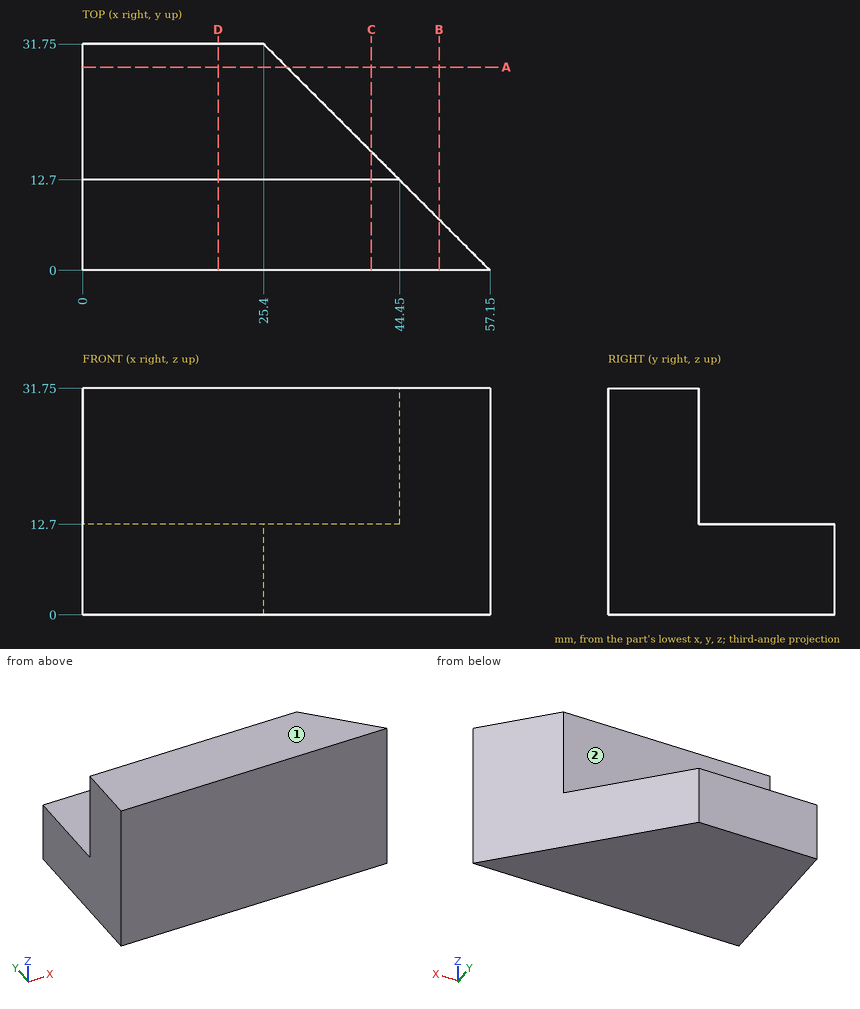
Can you work these out from the drawing? Everything is in mm from the part's minimum corner. A direction names the side the tool comes from. Coordinates: 2 decimals unless noted, no trailing zeros. Write each loop counter-clockwise with the first axis right and the second up, starting at its lowest first coordinate (ties: lowest second). Pieces come first, ordered by that corner, then holes. Notation, with made-up numbers: (-8.75, 32) -> (1.25, 32) arc R14 ccw to (1.25, 49) -> close; hole circle Ø11 at (76.5, -39.5). An arc over 180 degrees is marked (long way). Return JSON: item names as keys, results as strings.
(1) Imagine slicing it at B-B, the plane x = 50. Please give me the cut outline in (y, z), then the cut area to 3 significant figures.
Numbers:
{"outline": "(0, 0) -> (7.15, 0) -> (7.15, 31.75) -> (0, 31.75) -> close", "area": "227 mm2"}
(2) I need wall thicknesses on L1, parallel to Z at x = 5, y = 13; L2, parallel to X at y = 12, z = 20. Which ranges of each line are inside material? Lowest first, please.
Numbers:
{"L1": "z = 0 to 12.7", "L2": "x = 0 to 45.15"}
(3) Imagine slicing it at C-C, the plane x = 40.5. Please give me the cut outline in (y, z).
Numbers:
{"outline": "(0, 0) -> (16.65, 0) -> (16.65, 12.7) -> (12.7, 12.7) -> (12.7, 31.75) -> (0, 31.75) -> close"}
(4) Which directions (+Z, -Z, +X, -X, +Y, -Y) give clear straight access to the entire face, cutting with the end or side of a thin tool? Please do the marked faces 1 and 2.
Numbers:
{"face 1": "+Z, +X, -X, +Y, -Y", "face 2": "+Z, +X, -X, +Y"}
(5) I'm going to push flat-ended pins straight in: pin 1 (6 mm diameter, centred on y = 12.5, z = 14.5, fed in from +X); pin 2 (9.5 mm diameter, centred on x = 22, y = 17.5, fed in from +Z). Where does each tip first touch, or does it pass through?
Numbers:
{"pin 1": "stops at x = 47.65", "pin 2": "stops at z = 12.7"}
(6) Imagine slicing it at D-D, the plane x = 19. Please give me the cut outline in (y, z).
Numbers:
{"outline": "(0, 0) -> (31.75, 0) -> (31.75, 12.7) -> (12.7, 12.7) -> (12.7, 31.75) -> (0, 31.75) -> close"}
(7) Imagine slicing it at A-A, the plane y = 28.5. Please give me the cut outline in (x, z).
Numbers:
{"outline": "(0, 0) -> (28.65, 0) -> (28.65, 12.7) -> (0, 12.7) -> close"}
